Job drawing, mm, ordinate dimensions from the low corner. One solid piece. Give positions to 0.01 mm unless a question says otherwise; leave off trailing zeros. Order: outer loops, then holes, each group sorted by start corner. A loop starts at its lowest first (then second) coordinate and runs counter-clockwise, first axis right, second up.
1. Slice it at C-C on x = 4. List the corners of the cut face in (y, z).
2. Drop flat-ended pins along their axis: pin 1 Ø4.5 at (y, z) = (30, 6.5) entering from +X; pin 2 Ø4.5 at (x, z) = (28.5, 3) entering from +Y. Give the stop position or say it passes through.
3. Probe line 1 (Y direction, x = 14.5, z = 5); line 2 (X direction, y = 45.5, z = 3.5). List the from-to ranges inside material, lowest first.
4. Slice it at B-B on y = 37.5. List the corners of the cut face in (x, z), and give its area (3 significant figures).
5. Slice it at A-A on z = 4.25. List the corners of the cut face in (x, y).
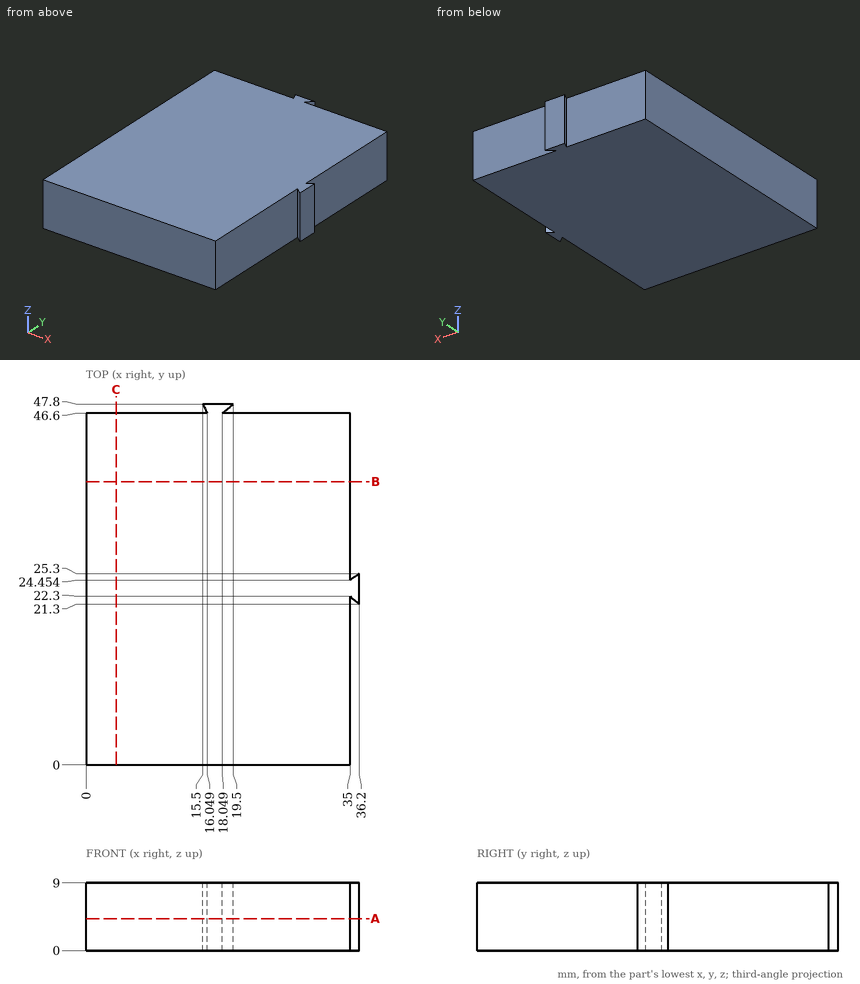
Data:
1. outline: (0, 0) - (46.6, 0) - (46.6, 9) - (0, 9) - close
2. pin 1: stops at x = 35
2. pin 2: stops at y = 46.6
3. line 1: y = 0 to 46.6
3. line 2: x = 0 to 35
4. outline: (0, 0) - (35, 0) - (35, 9) - (0, 9) - close
4. area: 315 mm2
5. outline: (0, 0) - (35, 0) - (35, 22.3) - (36.2, 21.3) - (36.2, 25.3) - (35, 24.45) - (35, 46.6) - (18.05, 46.6) - (19.5, 47.8) - (15.5, 47.8) - (16.05, 46.6) - (0, 46.6) - close
